```python
from build123d import *

# Parameters (mm, degrees)
F1_DEPTH  = 0.5
F0_W      = 328.2
F0_H      = 8.5
F2_DEPTH  = 0.8
F0_W_2    = 330
F0_H_2    = 71.4
F3_DEPTH  = 6.7
F0_W_3    = 0.6
F0_H_3    = 60.3
F4_DEPTH  = 5
F6_DEPTH  = 5.9
F7_W      = 18.5
F7_H      = 2.7
F8_DEPTH  = 0.9
F9_R      = 0.75
F10_W     = 0.6
F10_H     = 1.5
F11_DEPTH = 5
F10_H_2   = 3
F12_DEPTH = 3
F13_R     = 1
F14_W     = 1.5
F14_H     = 0.4
F15_DEPTH = 0.6
F16_R     = 0.25


with BuildPart() as f1:
    # F0 (on Top) → F1 (new body)
    with BuildSketch(Plane.XY):
        Polygon((-164.1, 34.8), (-164.1, -26.3), (164.1, -26.3), (164.1, 34.8), (109.9, 34.8), (109.9, -25.5), (109.3, -25.5), (109.3, 34.8), (55.1, 34.8), (55.1, -25.5), (54.5, -25.5), (54.5, 34.8), (0.3, 34.8), (0.3, -25.5), (-0.3, -25.5), (-0.3, 34.8), (-54.5, 34.8), (-54.5, -25.5), (-55.1, -25.5), (-55.1, 34.8), (-109.3, 34.8), (-109.3, -25.5), (-109.9, -25.5), (-109.9, 34.8), align=None)
        with BuildLine():
            ThreePointArc((-156, 22.7), (-154.8284271247, 25.5284271247), (-152, 26.7))
            Line((-152, 26.7), (-122, 26.7))
            ThreePointArc((-122, 26.7), (-119.1715728753, 25.5284271247), (-118, 22.7))
            Line((-118, 22.7), (-118, -13.3))
            ThreePointArc((-118, -13.3), (-119.1715728753, -16.1284271247), (-122, -17.3))
            Line((-122, -17.3), (-152, -17.3))
            ThreePointArc((-152, -17.3), (-154.8284271247, -16.1284271247), (-156, -13.3))
            Line((-156, -13.3), (-156, 22.7))
        make_face(mode=Mode.SUBTRACT)
        with BuildLine():
            ThreePointArc((-67.2, 26.7), (-64.3715728753, 25.5284271247), (-63.2, 22.7))
            Line((-63.2, 22.7), (-63.2, -13.3))
            ThreePointArc((-63.2, -13.3), (-64.3715728753, -16.1284271247), (-67.2, -17.3))
            Line((-67.2, -17.3), (-97.2, -17.3))
            ThreePointArc((-97.2, -17.3), (-100.0284271247, -16.1284271247), (-101.2, -13.3))
            Line((-101.2, -13.3), (-101.2, 22.7))
            ThreePointArc((-101.2, 22.7), (-100.0284271247, 25.5284271247), (-97.2, 26.7))
            Line((-97.2, 26.7), (-67.2, 26.7))
        make_face(mode=Mode.SUBTRACT)
        with BuildLine():
            ThreePointArc((-12.4, 26.7), (-9.5715728753, 25.5284271247), (-8.4, 22.7))
            Line((-8.4, 22.7), (-8.4, -13.3))
            ThreePointArc((-8.4, -13.3), (-9.5715728753, -16.1284271247), (-12.4, -17.3))
            Line((-12.4, -17.3), (-42.4, -17.3))
            ThreePointArc((-42.4, -17.3), (-45.2284271247, -16.1284271247), (-46.4, -13.3))
            Line((-46.4, -13.3), (-46.4, 22.7))
            ThreePointArc((-46.4, 22.7), (-45.2284271247, 25.5284271247), (-42.4, 26.7))
            Line((-42.4, 26.7), (-12.4, 26.7))
        make_face(mode=Mode.SUBTRACT)
        with BuildLine():
            ThreePointArc((42.4, 26.7), (45.2284271247, 25.5284271247), (46.4, 22.7))
            Line((46.4, 22.7), (46.4, -13.3))
            ThreePointArc((46.4, -13.3), (45.2284271247, -16.1284271247), (42.4, -17.3))
            Line((42.4, -17.3), (12.4, -17.3))
            ThreePointArc((12.4, -17.3), (9.5715728753, -16.1284271247), (8.4, -13.3))
            Line((8.4, -13.3), (8.4, 22.7))
            ThreePointArc((8.4, 22.7), (9.5715728753, 25.5284271247), (12.4, 26.7))
            Line((12.4, 26.7), (42.4, 26.7))
        make_face(mode=Mode.SUBTRACT)
        with BuildLine():
            ThreePointArc((97.2, 26.7), (100.0284271247, 25.5284271247), (101.2, 22.7))
            Line((101.2, 22.7), (101.2, -13.3))
            ThreePointArc((101.2, -13.3), (100.0284271247, -16.1284271247), (97.2, -17.3))
            Line((97.2, -17.3), (67.2, -17.3))
            ThreePointArc((67.2, -17.3), (64.3715728753, -16.1284271247), (63.2, -13.3))
            Line((63.2, -13.3), (63.2, 22.7))
            ThreePointArc((63.2, 22.7), (64.3715728753, 25.5284271247), (67.2, 26.7))
            Line((67.2, 26.7), (97.2, 26.7))
        make_face(mode=Mode.SUBTRACT)
        with BuildLine():
            ThreePointArc((152, 26.7), (154.8284271247, 25.5284271247), (156, 22.7))
            Line((156, 22.7), (156, -13.3))
            ThreePointArc((156, -13.3), (154.8284271247, -16.1284271247), (152, -17.3))
            Line((152, -17.3), (122, -17.3))
            ThreePointArc((122, -17.3), (119.1715728753, -16.1284271247), (118, -13.3))
            Line((118, -13.3), (118, 22.7))
            ThreePointArc((118, 22.7), (119.1715728753, 25.5284271247), (122, 26.7))
            Line((122, 26.7), (152, 26.7))
        make_face(mode=Mode.SUBTRACT)
    extrude(amount=F1_DEPTH)

    # F0 (on Top) → F2 (join)
    with BuildSketch(Plane.XY):
        with Locations((0, -30.55)):
            Rectangle(F0_W, F0_H)
    extrude(amount=F2_DEPTH)

    # F0 (on Top) → F3 (join)
    with BuildSketch(Plane.XY):
        Rectangle(F0_W_2, F0_H_2)
        Polygon((164.1, -34.8), (-164.1, -34.8), (-164.1, -26.3), (-164.1, 34.8), (-109.9, 34.8), (-109.3, 34.8), (-55.1, 34.8), (-54.5, 34.8), (-0.3, 34.8), (0.3, 34.8), (54.5, 34.8), (55.1, 34.8), (109.3, 34.8), (109.9, 34.8), (164.1, 34.8), (164.1, -26.3), align=None, mode=Mode.SUBTRACT)
    extrude(amount=F3_DEPTH)

    # F0 (on Top) → F4 (join)
    with BuildSketch(Plane.XY):
        with Locations((-109.6, 4.65)):
            Rectangle(F0_W_3, F0_H_3)
        with Locations((-54.8, 4.65)):
            Rectangle(F0_W_3, F0_H_3)
        with Locations((0, 4.65)):
            Rectangle(F0_W_3, F0_H_3)
        with Locations((54.8, 4.65)):
            Rectangle(F0_W_3, F0_H_3)
        with Locations((109.6, 4.65)):
            Rectangle(F0_W_3, F0_H_3)
    extrude(amount=F4_DEPTH)

    # F5 (on face) → F6 (join, through all)
    with BuildSketch(Plane.XY.offset(0.8)):
        with BuildLine():
            Line((-163.6753737487, -29.2), (-164.1, -29.2))
            Line((-164.1, -29.2), (-164.1, -34.8))
            Line((-164.1, -34.8), (-163.5, -34.8))
            Line((-163.5, -34.8), (-163.5, -29.3753737487))
            ThreePointArc((-163.5, -29.3753737487), (-163.5513657817, -29.2513657817), (-163.6753737487, -29.2))
        make_face()
    extrude(amount=F6_DEPTH)

    # F7 (on face) → F8 (cut, through all)
    with BuildSketch(Plane.XZ.offset(35.7)):
        with Locations((-128.75, 5.35)):
            Rectangle(F7_W, F7_H)
    extrude(amount=-F8_DEPTH, mode=Mode.SUBTRACT)

    # F9
    f9_edges = [f1.edges().sort_by_distance(p)[0] for p in [
        (-138, -35.25, 6.7),
        (-119.5, -35.25, 6.7),
        (-138, -35.25, 4),
        (-119.5, -35.25, 4),
    ]]
    fillet(f9_edges, radius=F9_R)

    # F10 (on face) → F11 (join)
    with BuildSketch(Plane.XY.offset(0.8)):
        with Locations((-138.4, -34.05)):
            Rectangle(F10_W, F10_H)
    extrude(amount=F11_DEPTH)

    # F10 (on face) → F12 (join)
    with BuildSketch(Plane.XY.offset(0.8)):
        with Locations((-93.8, -33.3)):
            Rectangle(F10_W, F10_H_2)
        with Locations((-58.2, -33.3)):
            Rectangle(F10_W, F10_H_2)
        with Locations((-49.2, -33.3)):
            Rectangle(F10_W, F10_H_2)
        with Locations((-13.3, -33.3)):
            Rectangle(F10_W, F10_H_2)
        with Locations((1.6, -33.3)):
            Rectangle(F10_W, F10_H_2)
        with Locations((58.7, -33.3)):
            Rectangle(F10_W, F10_H_2)
    extrude(amount=F12_DEPTH)

    # F13
    f13_edges = [f1.edges().sort_by_distance(p)[0] for p in [
        (58.7, -31.8, 3.8),
        (1.6, -31.8, 3.8),
        (-13.3, -31.8, 3.8),
        (-49.2, -31.8, 3.8),
        (-58.2, -31.8, 3.8),
        (-93.8, -31.8, 3.8),
    ]]
    fillet(f13_edges, radius=F13_R)

    # F14 (on face) → F15 (join)
    with BuildSketch(Plane(origin=(-138.7, 0, 0), x_dir=(0, -1, 0), z_dir=(-1, 0, 0))):
        with Locations((34.05, 5.6)):
            Rectangle(F14_W, F14_H)
    extrude(amount=F15_DEPTH)

    # F16
    f16_edges = [f1.edges().sort_by_distance(p)[0] for p in [
        (-138.1, -34.05, 5.8),
    ]]
    fillet(f16_edges, radius=F16_R)


solid = f1.part
```
Input: part model. Units: mm. Frame: model coordinates. A direction names the side the tool comes from. Coordinates: 2 decimals unless noted, no trailing zeros. Loops run counter-clockwise (first coordinate to the right, second up) from the corner with the lowest first, then second, coordinate; pieces in that order, holes last.
Q1. Line query: line 1 along Y through (x, z) = (-47, 6); line 2 along X through (y, z) = (-1, 6); line 3 along Z through (x, y) = (-68.5, -33). Output: solid intervals per line, ascending.
Results are:
line 1: y = -35.7 to -34.8, 34.8 to 35.7
line 2: x = -165 to -164.1, 164.1 to 165
line 3: z = 0 to 0.8
Q2. Section A-A, the plane x = 134.5. Return the cut outline in (y, z).
Results are:
outline: (-35.7, 0) - (-17.3, 0) - (-17.3, 0.5) - (-26.3, 0.5) - (-26.3, 0.8) - (-34.8, 0.8) - (-34.8, 6.7) - (-35.7, 6.7) - close; (26.7, 0) - (35.7, 0) - (35.7, 6.7) - (34.8, 6.7) - (34.8, 0.5) - (26.7, 0.5) - close
Q3. Set-up query: faces 5 (the flat face through (164.1, 0, 4)), 6 (the flat face through (165, 0, 3)). Return all of +Z, -Z, +X, -X, +Y, -Y with unobstructed straight access to the full face (end or side cutting, diameter ignored); none if empty.
Results are:
face 5: +Z
face 6: +Z, -Z, +X, +Y, -Y
Q4. Contact query for flat-ended pins moving along their axis: pin 1 (0.5 mm diameter, centred on x = 0, y = 16.5, fed in from +Z); pin 2 (10 mm diameter, centred on x = -66.5, y = -20.5, fed in from +Z); pin 3 (0.5 mm diameter, centred on x = -94, y = -33.5, fed in from +Z). Output: stop coordinate, or through.
Results are:
pin 1: stops at z = 5
pin 2: stops at z = 0.5
pin 3: stops at z = 3.8
Q5. Mould query, pull axis X, two halves, no side actions, for faces 1 (the flat face through (-2, 5, 0.5)), 2 (the flat face through (-165, 0, 3)), 3 (the flat face through (-2, -30, 0.8)), 4 (the flat face through (-2, 35.7, 3)). Classes: +X half, -X half, draft (parallel to the pull), parting line (faces both ways), or undercut.
Results are:
face 1: undercut
face 2: -X half
face 3: undercut
face 4: draft
Q6. Section C-C, the plane y = 2. Give the number of separate pieces and of enclosed holes in the cut face, and give its area (3 significant figures).
Results are:
separate pieces: 7
enclosed holes: 0
area: 75.7 mm2
Q7. Section B-B, the plane y = 31.5. Return the cut outline in (x, z).
Results are:
outline: (-165, 0) - (165, 0) - (165, 6.7) - (164.1, 6.7) - (164.1, 0.5) - (109.9, 0.5) - (109.9, 5) - (109.3, 5) - (109.3, 0.5) - (55.1, 0.5) - (55.1, 5) - (54.5, 5) - (54.5, 0.5) - (0.3, 0.5) - (0.3, 5) - (-0.3, 5) - (-0.3, 0.5) - (-54.5, 0.5) - (-54.5, 5) - (-55.1, 5) - (-55.1, 0.5) - (-109.3, 0.5) - (-109.3, 5) - (-109.9, 5) - (-109.9, 0.5) - (-164.1, 0.5) - (-164.1, 6.7) - (-165, 6.7) - close
